Build history of the part. All positions in model axes, mm. Round coordinates to 2 decimals unless told otherwise and drop trailing zeros. Write each loop counter-clockwise with the first axis right and the second up, starting at its lowest first coordinate (ties: lowest second). Pieces come first, ordered by that corner, then holes. Notation, with made-up numbers: M -1.5,36 L 46.5,36 A17 cw 46.5,51 Z; hole C -4,-3.5 d7. An arc over 180 degrees is marked long. Write item = value, one per line.
from build123d import *

# Parameters (mm, degrees)
ESBO_O1_R          = 22.5
FLANGE_BASE1_DEPTH = 12.7


# Sheet-metal steps are written as plain solids
with BuildPart() as part:
    # Esboço1 → Flange-base1 (new body)
    with BuildSketch(Plane(origin=(0, 0, 0), x_dir=(1, 0, 0), z_dir=(0, 1, 0))):
        with BuildLine():
            Line((-40, 0), (40, 0))
            Line((40, 0), (40, 80.7))
            ThreePointArc((40, 80.7), (0, 120.7), (-40, 80.7))
            Line((-40, 80.7), (-40, 0))
        make_face()
        with Locations(Location((0, 80.7, 0), (0, 0, 270))):
            Circle(ESBO_O1_R, mode=Mode.SUBTRACT)
    extrude(amount=-FLANGE_BASE1_DEPTH)


solid = part.part
1. Flat gauge pin, fed straight in: pin 1 (1.5 mm diameter, centred on y = -2.5, z = -106, fed in from +X). Where does the tip first touch, or does it go through?
Responses:
pin_1 = 31.58
2. Mould opens along Z. For faces 1 (the face through (-40, -6, -41)), 2 (the face through (-1, -6, 0)), 3 (the face through (0.88, -6.26, -120.69)), 4 (the face through (-8.618, -6.261, -59.916)) say: pulls with the +Z half, pulls with the -Z half, needs draft (parallel to the pull), parting line crosses it, or undercut.
Responses:
face_1 = needs draft
face_2 = pulls with the +Z half
face_3 = pulls with the -Z half
face_4 = undercut
3. Band-saw the part on D-D (z = -105.5). List the corners of the cut face in (x, y), plus the area to 3 significant figures.
Responses:
outline = M -31.38,-12.7 L 31.38,-12.7 L 31.38,0 L -31.38,0 Z
area = 797 mm²
4. Band-saw the part on C-C (y = -6.75). List the corners of the cut face in (x, z), plus the area to 3 significant figures.
Responses:
outline = M -40,-80.7 A40 ccw 40,-80.7 L 40,0 L -40,0 Z; hole C 0,-80.7 d45
area = 7,380 mm²
5. Band-saw the part on A-A (x = 0). List the corners of the cut face in (y, z).
Responses:
outline = M -12.7,-120.7 L 0,-120.7 L 0,-103.2 L -12.7,-103.2 Z; M -12.7,-58.2 L 0,-58.2 L 0,0 L -12.7,0 Z
6. Band-saw the part on B-B (z = -78). List the corners of the cut face in (x, y).
Responses:
outline = M -40,-12.7 L -22.34,-12.7 L -22.34,0 L -40,0 Z; M 22.34,-12.7 L 40,-12.7 L 40,0 L 22.34,0 Z
7. Probe probe 1 along X at (y, z) = (-2.75, -80.7); probe 2 along Z at (x, y) = (-8.5, -7.5); probe 3 along X at (y, z) = (-10, -95.5). List the from-to ranges inside material, lowest first.
Responses:
probe_1 = -40 to -22.5, 22.5 to 40
probe_2 = -119.79 to -101.53, -59.87 to 0
probe_3 = -37.16 to -16.95, 16.95 to 37.16
